Build history of the part. All positions in model axes, mm. Give positions to 0.01 mm unless a question says otherwise; leave off trailing zeros. Order: outer loops, then holes, each group sorted by start corner. A loop starts at its lowest first (then second) coordinate and runs counter-clockwise, first axis right, second up. Notation, with made-up numbers: M -38,77 L -28,77 A19 cw -28,107 Z; hole C -24,-12.5 d11. An arc over 180 degrees is marked long. One line per item, written item: value.
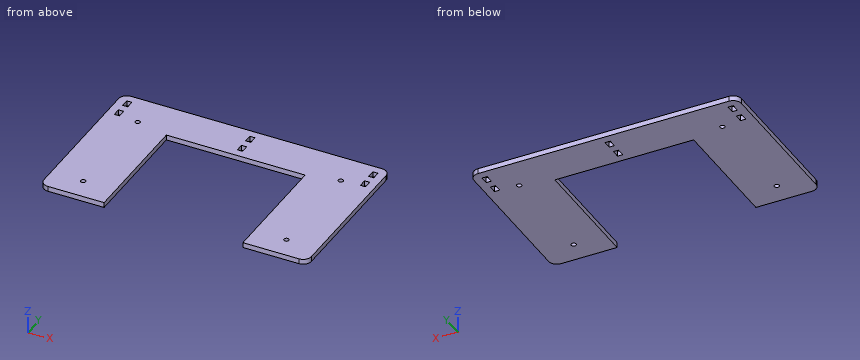
from build123d import *

# Parameters (mm, degrees)
F0_W      = 166
F0_H      = 100
F1_DEPTH  = 3.2
F2_R      = 5
F3_R      = 1.5
F4_DEPTH  = 25
F6_DEPTH  = 25
F7_W      = 3.2
F7_H      = 5
F8_DEPTH  = 25
F9_W      = 86.2
F9_H      = 5
F10_DEPTH = 3.2
F11_W     = 3.2
F11_H     = 5
F12_DEPTH = 25


with BuildPart() as f1:
    # F0 (on Top) → F1 (new body)
    with BuildSketch(Plane.XY):
        Rectangle(F0_W, F0_H)
    extrude(amount=F1_DEPTH)

    # F2
    f2_edges = [f1.edges().sort_by_distance(p)[0] for p in [
        (83, 50, 1.6),
        (83, -50, 1.6),
        (-83, -50, 1.6),
        (-83, 50, 1.6),
    ]]
    fillet(f2_edges, radius=F2_R)

    # F3 (on face) → F4 (cut)
    with BuildSketch(Plane.XY.offset(3.2)):
        with Locations((63.1, 29.2)):
            Circle(F3_R)
        with Locations((-63.1, 29.2)):
            Circle(F3_R)
        with Locations((-63.1, -36.45)):
            Circle(F3_R)
        with Locations((63.1, -36.45)):
            Circle(F3_R)
    extrude(amount=-F4_DEPTH, mode=Mode.SUBTRACT)

    # F5 (on face) → F6 (cut)
    with BuildSketch(Plane.XY.offset(3.2)):
        Polygon((43.1, 30), (0, 30), (-43.1, 30), (-43.1, -50), (43.1, -50), align=None)
    extrude(amount=-F6_DEPTH, mode=Mode.SUBTRACT)

    # F7 (on face) → F8 (cut)
    with BuildSketch(Plane.XY.offset(3.2)):
        with Locations((-76.4, 42.5)):
            Rectangle(F7_W, F7_H)
        with Locations((-76.4, 32.5)):
            Rectangle(F7_W, F7_H)
        with Locations((76.4, 32.5)):
            Rectangle(F7_W, F7_H)
        with Locations((76.4, 42.5)):
            Rectangle(F7_W, F7_H)
    extrude(amount=-F8_DEPTH, mode=Mode.SUBTRACT)

    # F9 (on face) → F10 (join, through all)
    with BuildSketch(Plane.XY.offset(3.2)):
        with Locations((0, 27.5)):
            Rectangle(F9_W, F9_H)
    extrude(amount=-F10_DEPTH)

    # F11 (on face) → F12 (cut)
    with BuildSketch(Plane(origin=(0, 0, 0), x_dir=(1, 0, 0), z_dir=(0, 0, -1))):
        with Locations((0, -32.5)):
            Rectangle(F11_W, F11_H)
        with Locations((0, -42.5)):
            Rectangle(F11_W, F11_H)
    extrude(amount=-F12_DEPTH, mode=Mode.SUBTRACT)


solid = f1.part
1) Saw through at C-C, the plane z = 0.75. Give the number of separate pieces and of enclosed holes in the cut face, then the cut area to 3 significant figures.
Check values:
separate pieces: 1
enclosed holes: 10
area: 9,990 mm^2
2) Saw through at B-B, the plane x = -22.5. Write the cut outline in (y, z), then the cut area to 3 significant figures.
Check values:
outline: M 25,0 L 50,0 L 50,3.2 L 25,3.2 Z
area: 80.0 mm^2
3) Pin check, flat tips, straight feed: pin 1 (3.5 mm diameter, centred on x = -63.1, y = 29.2, fed in from -Z); pin 2 (1.6 mm diameter, centred on x = 0.5, z = 1.5, fed in from -Y). Stop position of each tip, or through.
Check values:
pin 1: z = 0
pin 2: y = 25
4) Saw through at A-A, the plane y = 3. Write the cut outline in (x, z).
Check values:
outline: M -83,0 L -43.1,0 L -43.1,3.2 L -83,3.2 Z; M 43.1,0 L 83,0 L 83,3.2 L 43.1,3.2 Z
5) Drill centre lines: probe 1 along Y at (x, z) = (63.1, 0.75); probe 2 along X at (y, z) = (9, 0.65); probe 3 along Y at (x, z) = (14, 2.45). Where is each one in solid material? Low to high. Write a range as from..to.
Check values:
probe 1: -50..-37.95, -34.95..27.7, 30.7..50
probe 2: -83..-43.1, 43.1..83
probe 3: 25..50
